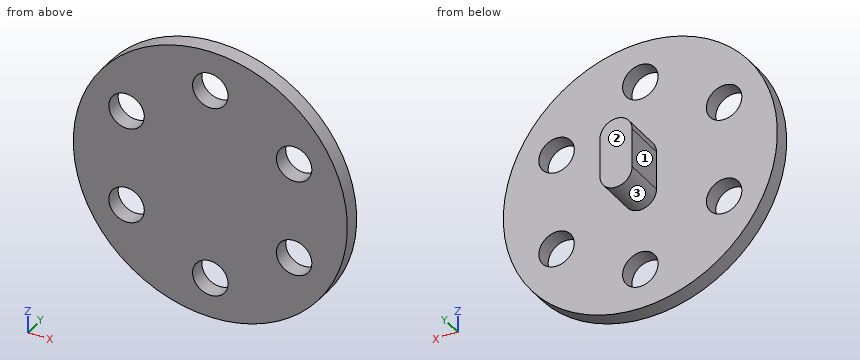
```python
from build123d import *

# Parameters (mm, degrees)
SKETCH1_R           = 42.5
SKETCH1_R_2         = 5.5
BOSS_EXTRUDE2_DEPTH = 5
BOSS_EXTRUDE3_DEPTH = 13


with BuildPart() as part:
    # Sketch1 → Boss-Extrude2 (new body)
    with BuildSketch(Plane(origin=(0, 0, 0), x_dir=(1, 0, 0), z_dir=(0, 1, 0))):
        with Locations(Location((0, 0, 0), (0, 0, 270))):
            Circle(SKETCH1_R)
        with Locations(Location((-25.980762114, 15, 0), (0, 0, 270))):
            Circle(SKETCH1_R_2, mode=Mode.SUBTRACT)
        with Locations(Location((0, 30, 0), (0, 0, 270))):
            Circle(SKETCH1_R_2, mode=Mode.SUBTRACT)
        with Locations(Location((25.980762114, 15, 0), (0, 0, 270))):
            Circle(SKETCH1_R_2, mode=Mode.SUBTRACT)
        with Locations(Location((25.980762114, -15, 0), (0, 0, 270))):
            Circle(SKETCH1_R_2, mode=Mode.SUBTRACT)
        with Locations(Location((0, -30, 0), (0, 0, 270))):
            Circle(SKETCH1_R_2, mode=Mode.SUBTRACT)
        with Locations(Location((-25.980762114, -15, 0), (0, 0, 270))):
            Circle(SKETCH1_R_2, mode=Mode.SUBTRACT)
    extrude(amount=BOSS_EXTRUDE2_DEPTH)

    # Sketch2 → Boss-Extrude3 (add)
    with BuildSketch(Plane(origin=(0, 5, 0), x_dir=(1, 0, 0), z_dir=(0, 1, 0))):
        with BuildLine():
            Line((-5, -6), (-5, 6))
            ThreePointArc((-5, 6), (0, 11), (5, 6))
            Line((5, 6), (5, -6))
            ThreePointArc((5, -6), (0, -11), (-5, -6))
        make_face()
    extrude(amount=BOSS_EXTRUDE3_DEPTH)


solid = part.part
```
Geometry check sheet. Reference: the model listing, model coordinates, mm. Face numbers are marked on the shaded views. A direction names the side the tool comes from. Coordinates: 2 decimals unless noted, no trailing zeros. Loops run counter-clockwise (first coordinate to the right, second up) from the corner with the lowest first, then second, coordinate; pieces in that order, holes last. Notation, with made-up numbers: (-16, 43) - (35, 43) arc R16 ccw to (35, 71) - close; hole circle Ø2 at (-32, -1.75). An arc over 180 degrees is marked (long way). One line per item, written item: value. Start each with the question number.
(1) Cross-section at C-C on z = 30. Enter the section's corners in (x, y).
(2) Cross-section at B-B on z = 13.5. Enter the section's corners in (x, y).
(3) Depth check by flat-ended pin: P1, Ø1.5, axis at y = 5.5, z = -30, coming from the -X side; P2, Ø6, axis at y = 4, z = 10, coming from the +X side; P3, Ø3, axis at x = 28, z = -7, coming from the -Y side; P4, Ø6.5, axis at x = -25.98, z = -15, coming from the +Y side. Enter the tip coordinate at first touch or a pass-through.
(4) Tool access check on the marked faces 1, 2 and 3. Record the directions out of +Z, -Z, +X, -X, +Y, -Y that give a thin tool (end or side, any length) a straight path to the whole face; none if there is none.
(5) Cross-section at A-A on x = 0. Enter the section's corners in (y, z).
(6) Cross-section at D-D on y = 2.25. Enter the section's corners in (x, z).
(7) Material ranges on line 1 (X direction, y = 2, z = 10.5); line 2 (X direction, y = 2.65, z = 15); line 3 (X direction, y = 6.25, z = -3.5), recorded low to high. Write a range as [from, to].
Results below:
1. outline: (-30.1, 0) - (-5.5, 0) - (-5.5, 5) - (-30.1, 5) - close; (5.5, 0) - (30.1, 0) - (30.1, 5) - (5.5, 5) - close
2. outline: (-40.3, 0) - (-31.27, 0) - (-31.27, 5) - (-40.3, 5) - close; (-20.69, 0) - (20.69, 0) - (20.69, 5) - (-20.69, 5) - close; (31.27, 0) - (40.3, 0) - (40.3, 5) - (31.27, 5) - close
3. P1: stops at x = -30.65
3. P2: stops at x = 41.92
3. P3: stops at y = 0
3. P4: passes through
4. face 1: +Z, -Z, -X, +Y
4. face 2: +Z, -Z, +X, -X, +Y
4. face 3: -Z, +Y
5. outline: (0, -42.5) - (5, -42.5) - (5, -35.5) - (0, -35.5) - close; (0, -24.5) - (5, -24.5) - (5, -11) - (18, -11) - (18, 11) - (5, 11) - (5, 24.5) - (0, 24.5) - close; (0, 35.5) - (5, 35.5) - (5, 42.5) - (0, 42.5) - close
6. outline: circle Ø85 at (0, 0); hole circle Ø11 at (-25.98, -15); hole circle Ø11 at (-25.98, 15); hole circle Ø11 at (0, -30); hole circle Ø11 at (0, 30); hole circle Ø11 at (25.98, -15); hole circle Ø11 at (25.98, 15)
7. line 1: x = [-41.18, -29.14], [-22.82, 22.82], [29.14, 41.18]
7. line 2: x = [-39.76, -31.48], [-20.48, 20.48], [31.48, 39.76]
7. line 3: x = [-5, 5]
